Autodesk Inventor part; units mm, degrees
ref_plane "YZ Plane" through (0, 0, 0) normal (1, 0, 0) x (0, 1, 0)
ref_plane "XZ Plane" through (0, 0, 0) normal (0, 1, 0) x (-1, 0, 0)
ref_plane "XY Plane" through (0, 0, 0) normal (0, 0, 1) x (1, 0, 0)
sketch "Эскиз1" plane through (0, 0, 0) normal (0, 0, 1) x (1, 0, 0)
  line L0 (-3.1, 3.1) -> (3.1, 3.1)
  line L1 (3.1, 3.1) -> (3.1, -3.1)
  line L2 (3.1, -3.1) -> (-3.1, -3.1)
  line L3 (-3.1, -3.1) -> (-3.1, 3.1)
  line L4 (-3.1, 3.1) -> (3.1, -3.1) construction
  line L5 (3.1, 3.1) -> (-3.1, -3.1) construction
  point P0 (0, 0)
  dimension "d0" = 6.2
  dimension "d1" = 6.2
extrude "Выдавливание1" add sketch "Эскиз1" along normal blind 4.8
fillet "Сопряжение1" radius 0.8 3 edges at (3.1, 3.1, 2.4) (3.1, -3.1, 2.4) (-3.1, 3.1, 2.4)
chamfer "Фаска1" distance 1.3 angle 45 1 edges at (-3.1, -3.1, 2.4)
sketch "Эскиз2" plane through (0, 0, 4.8) normal (0, 0, 1) x (1, 0, 0)
  circle A0 centre (0, 0) radius 2.05
  circle A1 centre (0, 0) radius 2.15
  dimension "d9" = 4.3
extrude "Выдавливание2" cut sketch "Эскиз2" against normal blind 4 contours A0 | A1
sketch "Эскиз3" plane through (0, 0, 0.8) normal (0, 0, 1) x (1, 0, 0)
  circle A0 centre (0, 0) radius 2.05
  dimension "d12" = 4.1
extrude "Выдавливание3" add sketch "Эскиз3" along normal blind 4
sketch "Эскиз4" plane through (0, 0, 4.8) normal (0, 0, 1) x (1, 0, 0)
  circle A0 centre (0, 0) radius 1.4
  dimension "d15" = 2.8
extrude "Выдавливание4" add sketch "Эскиз4" along normal blind 0.1
sketch "Эскиз5" plane through (0, 0, 0) normal (0, 0, -1) x (-1, 0, 0)
  line L0 (-1.6, -1) -> (-2.6, -1)
  line L1 (-2.6, -1) -> (-2.6, 1)
  line L2 (-2.6, 1) -> (-1.6, 1)
  line L3 (-1.6, 1) -> (-1.6, -1)
  line L4 (-1.6, -1) -> (-2.6, 1) construction
  line L5 (-2.6, -1) -> (-1.6, 1) construction
  line L6 (1.6, -1) -> (2.6, -1)
  line L7 (2.6, -1) -> (2.6, 1)
  line L8 (2.6, 1) -> (1.6, 1)
  line L9 (1.6, 1) -> (1.6, -1)
  line L10 (1.6, -1) -> (2.6, 1) construction
  line L11 (2.6, -1) -> (1.6, 1) construction
  point P0 (0, 0)
  dimension "d28" = 1
  dimension "d29" = 2
  dimension "d31" = 1
  dimension "d32" = 2
extrude "Выдавливание5" add sketch "Эскиз5" along normal blind 0.1
Can you work these out from the model? Positions are in its coordinate system, mm. A direction names the side the tool comes from. Coordinates: 2 decimals unless noted, no trailing zeros. Order: outer loops, then holes, each group sorted by start corner. A loop starts at its lowest first (then second) coordinate and runs counter-clockwise, first axis right, second up. Notation, with made-up numbers: (-16.5, 44) - (-5.5, 44) arc R26 ccw to (-5.5, 62) - close; hole circle Ø6 at (38.5, 87). An arc over 180 degrees is marked (long way). Answer in a Markdown table with one row per item.
1. For pin 1 (1.9 mm diameter, centred on x = 0, y = 0, fed in from -Z), with a flat end and sliding along its axis, tell me the tip position at first contact or that it passes through.
Reply:
| item | result |
|---|---|
| pin 1 | stops at z = 0 |
2. Suppose I cut it at D-D (z = 0.45). Please give me the cut outline in (x, y).
Reply:
| item | result |
|---|---|
| outline | (-3.1, -1.8) - (-1.8, -3.1) - (2.3, -3.1) arc R0.8 ccw to (3.1, -2.3) - (3.1, 2.3) arc R0.8 ccw to (2.3, 3.1) - (-2.3, 3.1) arc R0.8 ccw to (-3.1, 2.3) - close |
3. Suppose I cut it at C-C (y = 0). Please give me the cut outline in (x, z).
Reply:
| item | result |
|---|---|
| outline | (-3.1, 0) - (-2.6, 0) - (-2.6, -0.1) - (-1.6, -0.1) - (-1.6, 0) - (1.6, 0) - (1.6, -0.1) - (2.6, -0.1) - (2.6, 0) - (3.1, 0) - (3.1, 4.8) - (2.15, 4.8) - (2.15, 0.8) - (2.05, 0.8) - (2.05, 4.8) - (1.4, 4.8) - (1.4, 4.9) - (-1.4, 4.9) - (-1.4, 4.8) - (-2.05, 4.8) - (-2.05, 0.8) - (-2.15, 0.8) - (-2.15, 4.8) - (-3.1, 4.8) - close |
4. If I drill on line 1 along Y through (x, z) = (1.75, 3.25); line 2 along Z through (x, y) = (1.25, 2); line 3 along Z through (x, y) = (-2, -0.25), over which ranges is the centre line in solid material (lowest first)?
Reply:
| item | result |
|---|---|
| line 1 | y = -3.1 to -1.25, -1.07 to 1.07, 1.25 to 3.1 |
| line 2 | z = 0 to 4.8 |
| line 3 | z = -0.1 to 4.8 |
5. For faces 1 (the flat face through (0, 3.1, 2)), 2 (the flat face through (0.9, -1.3, 4.8)), which set-ups out of +Z, -Z, +X, -X, +Y, -Y let a thin tool reach every point of the face, with its end or its side?
Reply:
| item | result |
|---|---|
| face 1 | +Z, -Z, +X, -X, +Y |
| face 2 | +Z |
6. Suppose I cut it at A-A (z = 3.8). Please give me the cut outline in (x, y).
Reply:
| item | result |
|---|---|
| outline | (-3.1, -1.8) - (-1.8, -3.1) - (2.3, -3.1) arc R0.8 ccw to (3.1, -2.3) - (3.1, 2.3) arc R0.8 ccw to (2.3, 3.1) - (-2.3, 3.1) arc R0.8 ccw to (-3.1, 2.3) - close; circle Ø4.1 at (0, 0); hole circle Ø4.3 at (0, 0) |
7. Suppose I cut it at B-B (x = 0). Please give me the cut outline in (y, z).
Reply:
| item | result |
|---|---|
| outline | (-3.1, 0) - (3.1, 0) - (3.1, 4.8) - (2.15, 4.8) - (2.15, 0.8) - (2.05, 0.8) - (2.05, 4.8) - (1.4, 4.8) - (1.4, 4.9) - (-1.4, 4.9) - (-1.4, 4.8) - (-2.05, 4.8) - (-2.05, 0.8) - (-2.15, 0.8) - (-2.15, 4.8) - (-3.1, 4.8) - close |
